Model file for the job. Use its own axes, mm. Face numbers are marked on the shaded views. A direction names the side the tool comes from. Round coordinates to 2 decimals unless told otherwise and drop trailing zeros. Loops run counter-clockwise (first coordinate to the right, second up) from the corner with the lowest first, then second, coordinate; pieces in that order, holes last. Notation, with made-up numbers: (7.25, 65.25) - (59.25, 65.25) arc R23 cw to (59.25, 73.25) - close; hole circle Ø2 at (79, 87). An arc over 180 degrees is marked (long way). Answer as a JSON object with one key per item and string values.
Autodesk Inventor part; units mm, degrees
ref_plane "YZ Plane" through (0, 0, 0) normal (1, 0, 0) x (0, 1, 0)
ref_plane "XZ Plane" through (0, 0, 0) normal (0, 1, 0) x (-1, 0, 0)
ref_plane "XY Plane" through (0, 0, 0) normal (0, 0, 1) x (1, 0, 0)
sketch "Sketch1" plane through (0, 0, 0) normal (0, 0, 1) x (1, 0, 0)
  circle A0 centre (0, 0) radius 39
  circle A1 centre (0, 0) radius 42 construction
  circle A2 centre (0, 42) radius 3 construction
  circle A3 centre (0, 0) radius 37
  circle A4 centre (0, 0) radius 45
  circle A5 centre (0, 0) radius 64.5
  dimension "d5" = 84
  dimension "d0" = 78
  dimension "d6" = 6
  dimension "d14" = 74
  dimension "d15" = 90
  dimension "d16" = 129
extrude "Extrusion2" add sketch "Sketch1" along normal blind 5 contours A5
extrude "Extrusion3" add sketch "Sketch1" along normal blind 7 contours A4
sketch "Sketch2" plane through (0, 0, 0) normal (0, 0, -1) x (-1, 0, 0)
  circle A0 centre (0, 0) radius 55.5
  circle A1 centre (0, 55.5) radius 4
  dimension "d21" = 111
  dimension "d22" = 8
extrude "Extrusion4" cut sketch "Sketch2" against normal through all contours A1 A0 | A0 A1 picked at (-0.157, 54.1653) picked at (0.1387, 56.8154)
pattern_circular "Circular Pattern1" count 6 over 360 about axis through (0, 0, -10) along (0, 0, 1) of "Extrusion4"
thread "Thread1"
thread "Thread2"
thread "Thread3"
thread "Thread4"
thread "Thread5"
thread "Thread6"
properties part number "back" material "Aluminum 6061"
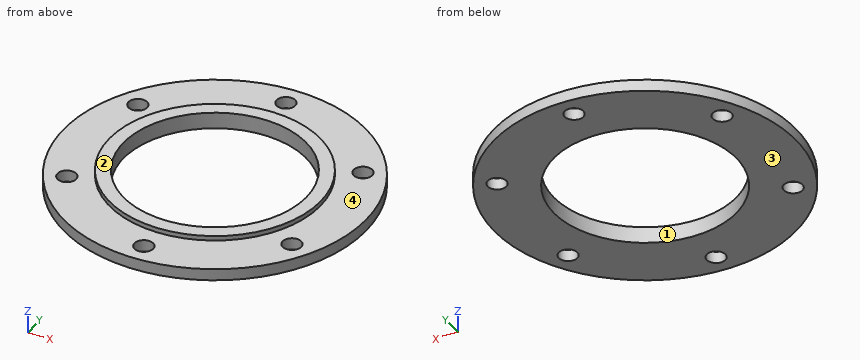
1) Tool access for the marked faces 3 and 4: list every direction of +Z, -Z, +X, -X, +Y, -Y with a clear straight run to the whole face (end or side of a thin tool).
Values follow:
{"face 3": "-Z, +X, -X, +Y, -Y", "face 4": "+Z"}
2) Slice it at B-B on y = 0. List the corners of the cut face in (x, z), then the cut area to 3 significant figures.
Values follow:
{"outline": "(-64.5, 0) - (-39, 0) - (-39, 7) - (-45, 7) - (-45, 5) - (-64.5, 5) - close; (39, 0) - (64.5, 0) - (64.5, 5) - (45, 5) - (45, 7) - (39, 7) - close", "area": "279 mm²"}
3) Two-plate mould, pull along X, no slides. Class the marked faces 1 and 2: pulls with the +X half, pulls with the -X half, needs draft (parallel to the pull), parting line crosses it, or undercut.
Values follow:
{"face 1": "undercut", "face 2": "needs draft"}
4) Slice it at D-D on x = -28.5. List the corners of the cut face in (y, z), then the cut area to 3 significant figures.
Values follow:
{"outline": "(-57.86, 0) - (-26.62, 0) - (-26.62, 7) - (-34.82, 7) - (-34.82, 5) - (-57.86, 5) - close; (26.62, 0) - (57.86, 0) - (57.86, 5) - (34.82, 5) - (34.82, 7) - (26.62, 7) - close", "area": "345 mm²"}
5) Slice it at A-A on x = 0. List the corners of the cut face in (y, z), then the cut area to 3 significant figures.
Values follow:
{"outline": "(-64.5, 0) - (-59.5, 0) - (-59.5, 5) - (-64.5, 5) - close; (-51.5, 0) - (-39, 0) - (-39, 7) - (-45, 7) - (-45, 5) - (-51.5, 5) - close; (39, 0) - (51.5, 0) - (51.5, 5) - (45, 5) - (45, 7) - (39, 7) - close; (59.5, 0) - (64.5, 0) - (64.5, 5) - (59.5, 5) - close", "area": "199 mm²"}
6) Probe probe 1 along Y at (x, z) = (0.5, 1.25); probe 2 along Y at (x, z) = (-1, 6.75); probe 3 along X at (y, z) = (-25, 4.25). List the from-to ranges inside material, lowest first.
Values follow:
{"probe 1": "-64.5 to -59.47, -51.53 to -39, 39 to 51.53, 59.47 to 64.5", "probe 2": "-44.99 to -38.99, 38.99 to 44.99", "probe 3": "-59.46 to -50.97, -45.16 to -29.93, 29.93 to 45.16, 50.97 to 59.46"}
7) Drop flat-ended pins along their axis: P1, Ø1.5, axis at x = 12.5, z = 6, coming from the +Y side; P2, Ø3, axis at x = 46.5, z = 3.5, coming from the +Y side; P3, Ø13, axis at x = 48.06, y = -27.75, coming from the +Z side. Give the stop position or say it passes through.
Values follow:
{"P1": "y = 43.44", "P2": "y = 46.21", "P3": "z = 5"}
8) Slice it at C-C on y = 27.75. List the corners of the cut face in (x, z).
Values follow:
{"outline": "(-58.23, 0) - (-52.06, 0) - (-52.06, 5) - (-58.23, 5) - close; (-44.06, 0) - (-27.4, 0) - (-27.4, 7) - (-35.43, 7) - (-35.43, 5) - (-44.06, 5) - close; (27.4, 0) - (44.06, 0) - (44.06, 5) - (35.43, 5) - (35.43, 7) - (27.4, 7) - close; (52.06, 0) - (58.23, 0) - (58.23, 5) - (52.06, 5) - close"}
